from build123d import *

# Parameters (mm, degrees)
F4_R     = 30.353
F6_DEPTH = 12.8524
F8_DEPTH = 25.4


with BuildPart() as f6:
    # F4 (on face) → F6 (new body)
    with BuildSketch(Plane.XY):
        with BuildLine():
            Line((-21.337585, -116.979506), (-21.337585, 147.294909))
            ThreePointArc((-21.337585, 147.294909), (-65.787585, 187.33966), (-110.237585, 147.294909))
            Line((-110.237585, 147.294909), (-110.237585, -167.779506))
            Line((-110.237585, -167.779506), (-21.337585, -116.979506))
        make_face()
        with Locations((-65.724085, 141.998894)):
            Circle(F4_R, mode=Mode.SUBTRACT)
    extrude(amount=F6_DEPTH)

    # F7 (on face) → F8 (cut)
    with BuildSketch(Plane.XY.offset(12.8524)):
        with BuildLine():
            ThreePointArc((-59.374085, 32.321694), (-61.233957, 36.811823), (-65.724085, 38.671694))
            ThreePointArc((-65.724085, 38.671694), (-70.214213, 27.831566), (-59.374085, 32.321694))
        make_face()
    extrude(amount=-F8_DEPTH, mode=Mode.SUBTRACT)


solid = f6.part
The model under review builds one solid part; all positions refer to its coordinate system, in mm. Round coordinates to 2 decimals unless told otherwise and drop trailing zeros. Loops run counter-clockwise (first coordinate to the right, second up) from the corner with the lowest first, then second, coordinate; pieces in that order, holes last. Notation, with made-up numbers: (15, 24) -> (56, 24) arc R28 cw to (56, 46) -> close; hole circle Ø11 at (36.25, 17). An arc over 180 degrees is marked (long way). Return JSON: item names as keys, results as strings.
(1) For pin 1 (6 mm diameter, centred on x = -43, z = 5, fed in from +Y); pin 2 (4 mm diameter, centred on x = -39, z = 8, fed in from -Y); pin 3 (5 mm diameter, centred on x = -97, z = 2.5, fed in from +Y), all flat-tipped, find the tip position at first contact; note any pin that passes through.
Solved:
{"pin 1": "y = 182.72", "pin 2": "y = -128.22", "pin 3": "y = 176.9"}
(2) Add section D-D on x = -27.5. Write out the cut boundary in (y, z), plus the area to 3 significant figures.
Solved:
{"outline": "(-120.5, 0) -> (165.7, 0) -> (165.7, 12.85) -> (-120.5, 12.85) -> close", "area": "3,680 mm2"}
(3) Add section C-C on x = -78.5. Write out the cut boundary in (y, z).
Solved:
{"outline": "(-149.64, 0) -> (114.47, 0) -> (114.47, 12.85) -> (-149.64, 12.85) -> close; (169.53, 0) -> (185.49, 0) -> (185.49, 12.85) -> (169.53, 12.85) -> close"}
(4) The part is to be moulded in two halves that separate along X. For faces 1 (the cylindrical face through (-49.406, 167.593, 6.336)), 2 (the flat face through (-66, 12, 12.852)), 3 (the flat face through (-21.338, 13, 6)), say which applies: released by +X, released by -X, zero draft, split by the parting line, or undercut.
Solved:
{"face 1": "undercut", "face 2": "zero draft", "face 3": "released by +X"}
(5) Add section B-B on z = 10. Write out the cut boundary in (x, y).
Solved:
{"outline": "(-110.24, -167.78) -> (-21.34, -116.98) -> (-21.34, 147.29) arc R44.69 ccw to (-110.24, 147.29) -> close; hole circle Ø60.71 at (-65.72, 142); hole (-65.72, 38.67) arc R6.35 ccw (long way) to (-59.37, 32.32) arc R6.35 ccw to start"}
(6) Add section A-A on x = -55.5. Write out the cut boundary in (y, z).
Solved:
{"outline": "(-136.5, 0) -> (113.42, 0) -> (113.42, 12.85) -> (-136.5, 12.85) -> close; (170.58, 0) -> (186.14, 0) -> (186.14, 12.85) -> (170.58, 12.85) -> close"}
(7) For line 1 (Y direction, x = -65, z = 2.25); line 2 (X direction, y = 38, z = 3.75); line 3 (X direction, y = 130.5, z = 6), list the stretches that pass through material, from the lowest coordinate up.
Solved:
{"line 1": "-141.93 to 26.01, 38.63 to 111.65, 172.34 to 187.33", "line 2": "-110.24 to -68.57, -62.88 to -21.34", "line 3": "-110.24 to -93.81, -37.63 to -21.34"}
